For this review, take the finished solid that the model builds, in its own axes (mm). Coordinates: 2 decimals unless noted, no trailing zeros. Loops run counter-clockwise (first coordinate to the right, second up) from the corner with the lowest first, then second, coordinate; pieces in that order, holes last.
1. Take a section at A-A, the plane x = -62. State the section outline as (y, z) points (3 decimals), then the cut area to 3 significant figures.
2. Take a section at C-C, the plane z = 0.75. Count the separate pieces of the cut face and the enclosed holes in it, then the cut area to 3 significant figures.
3. Take a section at B-B, the plane y = -3.5. State the section outline as (x, z) points (3 decimals), then the cut area to 3 significant figures.
4. Clearance check with flat-ended pins moving along their axes: P1, Ø4, axis at x = -10, y = 12.825, coming from the -Z side; P2, Ø22.5, axis at x = -62, y = 0, coming from the -Z side. State where each tip first meets the part, or that it passes through.
5. To check wall thickness, follow probe 1 along Y at (x, z) = (-54, 1.45); probe 2 along Y at (x, z) = (6, 1.35); probe 3 along Y at (x, z) = (-60, 2.25). State the ranges of each line that lie inside material, in increasing order.
6. Mouldability with a two-part tool opening along Y and no side actions: class faces 1 (the face through (-1, 0, 3.175)), 2 (the face through (-1, 24, 2)), 3 (the face through (-75.719, -21.594, 1.61)), 4 (the face through (5.443, 10.314, 1.61)) as pulls with the +Y half, pulls with the -Y half, needs draft (parallel to the pull), parting line crosses it, or undercut.
```python
from build123d import *

# Parameters (mm, degrees)
SKETCH2_W           = 156
SKETCH2_H           = 48
SKETCH2_R           = 2.05
SKETCH2_R_2         = 7.05
BOSS_EXTRUDE2_DEPTH = 3.175
FILLET1_R           = 8
SKETCH3_R           = 2.571717643
CUT_EXTRUDE1_DEPTH  = 10


with BuildPart() as part:
    # Sketch2 → Boss-Extrude2 (new body)
    with BuildSketch(Plane.XY):
        Rectangle(SKETCH2_W, SKETCH2_H)
        with Locations((-70, 8)):
            Circle(SKETCH2_R, mode=Mode.SUBTRACT)
        with Locations((-54, 8)):
            Circle(SKETCH2_R, mode=Mode.SUBTRACT)
        with Locations((-54, -8)):
            Circle(SKETCH2_R, mode=Mode.SUBTRACT)
        with Locations((-70, -8)):
            Circle(SKETCH2_R, mode=Mode.SUBTRACT)
        with Locations((-62, 0)):
            Circle(SKETCH2_R_2, mode=Mode.SUBTRACT)
    extrude(amount=BOSS_EXTRUDE2_DEPTH)

    # Fillet1
    fillet1_edges = [part.edges().sort_by_distance(p)[0] for p in [
        (78, 24, 1.5875),
        (78, -24, 1.5875),
        (-78, -24, 1.5875),
        (-78, 24, 1.5875),
    ]]
    fillet(fillet1_edges, radius=FILLET1_R)

    # Sketch3 → Cut-Extrude1 (cut)
    with BuildSketch(Plane.XY.offset(3.175)):
        with Locations((70, 12.825)):
            Circle(SKETCH3_R)
        with Locations((62, 12.825)):
            Circle(SKETCH3_R)
        with Locations((54, 12.825)):
            Circle(SKETCH3_R)
        with Locations((46, 12.825)):
            Circle(SKETCH3_R)
        with Locations((38, 12.825)):
            Circle(SKETCH3_R)
        with Locations((30, 12.825)):
            Circle(SKETCH3_R)
        with Locations((22, 12.825)):
            Circle(SKETCH3_R)
        with Locations((14, 12.825)):
            Circle(SKETCH3_R)
        with Locations((6, 12.825)):
            Circle(SKETCH3_R)
        with Locations((-2, 12.825)):
            Circle(SKETCH3_R)
        with Locations((-10, 12.825)):
            Circle(SKETCH3_R)
        with Locations((-18, 12.825)):
            Circle(SKETCH3_R)
    extrude(amount=-CUT_EXTRUDE1_DEPTH, mode=Mode.SUBTRACT)


solid = part.part
```
Results list:
1. outline: (-24, 0) - (-7.05, 0) - (-7.05, 3.175) - (-24, 3.175) - close; (7.05, 0) - (24, 0) - (24, 3.175) - (7.05, 3.175) - close
1. area: 108 mm2
2. separate pieces: 1
2. enclosed holes: 17
2. area: 6,970 mm2
3. outline: (-78, 0) - (-68.12, 0) - (-68.12, 3.175) - (-78, 3.175) - close; (-55.88, 0) - (78, 0) - (78, 3.175) - (-55.88, 3.175) - close
3. area: 456 mm2
4. P1: passes through
4. P2: stops at z = 0
5. probe 1: y = -24 to -10.05, -5.95 to 5.95, 10.05 to 24
5. probe 2: y = -24 to 10.25, 15.4 to 24
5. probe 3: y = -24 to -6.76, 6.76 to 24
6. face 1: needs draft
6. face 2: pulls with the +Y half
6. face 3: pulls with the -Y half
6. face 4: undercut
